from build123d import *

# Parameters (mm, degrees)
F0_W     = 190
F0_H     = 240
F1_DEPTH = 3
F2_W     = 190
F2_H     = 240
F2_W_2   = 184
F2_H_2   = 234
F3_DEPTH = 80
F4_W     = 60
F4_H     = 40
F5_DEPTH = 0.5
F6_W     = 60
F6_H     = 40
F7_DEPTH = 0.5


with BuildPart() as f1:
    # F0 (on Top) → F1 (new body)
    with BuildSketch(Plane.XY):
        with Locations((-3.855437, -43.830654)):
            Rectangle(F0_W, F0_H)
    extrude(amount=F1_DEPTH)

    # F2 (on face) → F3 (join)
    with BuildSketch(Plane.XY.offset(3)):
        with Locations((-3.855437, -43.830654)):
            Rectangle(F2_W, F2_H)
        with Locations((-3.855437, -43.830654)):
            Rectangle(F2_W_2, F2_H_2, mode=Mode.SUBTRACT)
    extrude(amount=F3_DEPTH)

    # F4 (on face) → F5 (cut)
    with BuildSketch(Plane(origin=(-98.855437, 0, 0), x_dir=(0, -1, 0), z_dir=(-1, 0, 0))):
        with Locations((-41.169346, 41.5)):
            Rectangle(F4_W, F4_H)
    extrude(amount=-F5_DEPTH, mode=Mode.SUBTRACT)

    # F6 (on face) → F7 (cut)
    with BuildSketch(Plane.YZ.offset(91.144563)):
        with Locations((41.169346, 41.5)):
            Rectangle(F6_W, F6_H)
    extrude(amount=-F7_DEPTH, mode=Mode.SUBTRACT)


solid = f1.part
Here's how the part is built. I have some questions about the finished solid (model axes, mm). A direction names the side the tool comes from. Give positions to 0.01 mm unless a question says otherwise; leave off trailing zeros. Order: outer loops, then holes, each group sorted by start corner. A loop starts at its lowest first (then second) coordinate and runs counter-clockwise, first axis right, second up. Notation, with made-up numbers: M 63.25,67 L 96.25,67 A18 cw 96.25,74 Z; hole C 41,-15.75 d10. An arc over 180 degrees is marked long. Answer as a JSON object with one key per item and string values. Group by question number.
1) Suppose I cut it at C-C, the plane y = 59. Write out the boundary of the cut face in (x, z), plus the area to 3 significant figures.
2) I'm going to push flat-ended pins straight in: pin 1 Ø12 at (y, z) = (52.5, 32.5) entering from +X; pin 2 Ø2 at (x, y) = (-16, 44.5) entering from +Z; pin 3 Ø1.5 at (y, z) = (21.5, 54.5) entering from -X. Where does each tip first touch, or does it pass through?
3) We'd pull the mould along Y, two halves only. Please class faces 4 (the flat face through (-98.855, -46, 41)), 5 (the flat face through (-5, 76.169, 41)), 6 (the flat face through (90.645, 41, 42)): pulls with the +Y half, pulls with the -Y half, needs draft (parallel to the pull), parting line crosses it, or undercut.
4) Suppose I cut it at B-B, the plane x = 4.5. Write out the boundary of the cut face in (y, z), plus the area to 3 significant figures.
5) Suppose I cut it at A-A, the plane z = 66. Write out the boundary of the cut face in (x, y).
6) On a 3-axis mill with a long thin cutter (end or side, diameter ignored), from which of +Z, -Z, +X, -X, +Y, -Y can I reach the whole of each face in a straight line? I mean faces 1 (the flat face through (-98.355, 42, 42)), 2 (the flat face through (-5, -160.831, 42)), 3 (the flat face through (-5, -163.831, 41)). Say none if no direction works.
7) Suppose I cut it at D-D, the plane z = 39. Write out the boundary of the cut face in (x, y).
8) Please list where these lines run through material, in increasing order: L1, parallel to X at y = -52, z = 78; L2, parallel to Y at x = -77.5, z = 65; L3, parallel to X at y = 44, z = 49. Write a range as [from, to].
Results found:
{
 "1": {"outline": "M -98.86,0 L 91.14,0 L 91.14,21.5 L 90.64,21.5 L 90.64,61.5 L 91.14,61.5 L 91.14,83 L 88.14,83 L 88.14,3 L -95.86,3 L -95.86,83 L -98.86,83 L -98.86,61.5 L -98.36,61.5 L -98.36,21.5 L -98.86,21.5 Z", "area": "1,010 mm²"},
 "2": {"pin 1": "x = 90.64", "pin 2": "z = 3", "pin 3": "x = -98.36"},
 "3": {"face 4": "needs draft", "face 5": "pulls with the +Y half", "face 6": "undercut"},
 "4": {"outline": "M -163.83,0 L 76.17,0 L 76.17,83 L 73.17,83 L 73.17,3 L -160.83,3 L -160.83,83 L -163.83,83 Z", "area": "1,200 mm²"},
 "5": {"outline": "M -98.86,-163.83 L 91.14,-163.83 L 91.14,76.17 L -98.86,76.17 Z; hole M -95.86,-160.83 L 88.14,-160.83 L 88.14,73.17 L -95.86,73.17 Z"},
 "6": {"face 1": "-X", "face 2": "+Z", "face 3": "+Z, -Z, +X, -X, -Y"},
 "7": {"outline": "M -98.86,-163.83 L 91.14,-163.83 L 91.14,11.17 L 90.64,11.17 L 90.64,71.17 L 91.14,71.17 L 91.14,76.17 L -98.86,76.17 L -98.86,71.17 L -98.36,71.17 L -98.36,11.17 L -98.86,11.17 Z; hole M -95.86,-160.83 L 88.14,-160.83 L 88.14,73.17 L -95.86,73.17 Z"},
 "8": {"L1": "[-98.86, -95.86], [88.14, 91.14]", "L2": "[-163.83, -160.83], [73.17, 76.17]", "L3": "[-98.36, -95.86], [88.14, 90.64]"}
}
